```python
from build123d import *

# Parameters (mm, degrees)
SKETCH1_R           = 1.375
BOSS_EXTRUDE1_DEPTH = 1.6
CUT_EXTRUDE1_DEPTH  = 0.1
SKETCH_1_W          = 13.191380008
SKETCH_1_H          = 13.254567414
EXTRUDE_1_DEPTH     = 8
SKETCH_2_W          = 10.236154205
SKETCH_2_H          = 10.074954926
EXTRUDE_2_DEPTH     = 8


with BuildPart() as part:
    # Sketch1 → Boss-Extrude1 (new body)
    with BuildSketch(Plane.XY):
        with BuildLine():
            Line((-39.5, -28), (39.5, -28))
            ThreePointArc((39.5, -28), (41.621320344, -27.121320344), (42.5, -25))
            Line((42.5, -25), (42.5, 25))
            ThreePointArc((42.5, 25), (41.621320344, 27.121320344), (39.5, 28))
            Line((39.5, 28), (-39.5, 28))
            ThreePointArc((-39.5, 28), (-41.621320344, 27.121320344), (-42.5, 25))
            Line((-42.5, 25), (-42.5, -25))
            ThreePointArc((-42.5, -25), (-41.621320344, -27.121320344), (-39.5, -28))
        make_face()
        with Locations((-39, 24.5)):
            Circle(SKETCH1_R, mode=Mode.SUBTRACT)
        with Locations((-39, -24.5)):
            Circle(SKETCH1_R, mode=Mode.SUBTRACT)
        with Locations((19, 24.5)):
            Circle(SKETCH1_R, mode=Mode.SUBTRACT)
        with Locations((19, -24.5)):
            Circle(SKETCH1_R, mode=Mode.SUBTRACT)
    extrude(amount=BOSS_EXTRUDE1_DEPTH)

    # Sketch2 → Cut-Extrude1 (cut)
    with BuildSketch(Plane.XY.offset(1.6)):
        Polygon((-35.65, -28.636850855), (-28.15, -28.636850855), (-28.15, -23.2), (-31.573707352, -23.2), (-31.573707352, -23.3), (-28.25, -23.3), (-28.25, -28.536850855), (-35.55, -28.536850855), (-35.55, -23.3), (-32.465045999, -23.3), (-32.465045999, -23.2), (-35.65, -23.2), align=None)
        Polygon((-17.75, -17.5), (-11.015830732, -17.5), (-11.015830732, -17.6), (-17.65, -17.6), (-17.65, -33.061376344), (-3.35, -33.061376344), (-3.35, -17.6), (-9.684859924, -17.6), (-9.684859924, -17.5), (-3.25, -17.5), (-3.25, -33.161376344), (-17.75, -33.161376344), align=None)
        Polygon((0.5, -5.3), (4.5, -5.3), (4.5, -27.7), (0.5, -27.7), (0.5, -17.125), (0.6, -17.125), (0.6, -27.6), (4.4, -27.6), (4.4, -5.4), (0.6, -5.4), (0.6, -15.17398131), (0.5, -15.17398131), align=None)
        Polygon((7.5, -15.5), (9.799158316, -15.5), (9.799158316, -15.6), (7.6, -15.6), (7.6, -31.061376344), (14.4, -31.061376344), (14.4, -15.6), (12.062610562, -15.6), (12.062610562, -15.5), (14.5, -15.5), (14.5, -31.161376344), (7.5, -31.161376344), align=None)
        Polygon((-35.45, 27), (15.45, 27), (15.45, 22), (-8.906687942, 22), (-8.906687942, 22.1), (15.35, 22.1), (15.35, 26.9), (-35.35, 26.9), (-35.35, 22.1), (-11.458179647, 22.1), (-11.458179647, 22), (-35.45, 22), align=None)
        Polygon((-41.371710411, -10.514157593), (-37.371710411, -10.514157593), (-37.371710411, 0.094714316), (-37.471710411, 0.094714316), (-37.471710411, -10.414157593), (-41.271710411, -10.414157593), (-41.271710411, 10.414157593), (-37.471710411, 10.414157593), (-37.471710411, 1), (-37.371710411, 1), (-37.371710411, 10.514157593), (-41.371710411, 10.514157593), align=None)
        Polygon((23.2, -25.5), (44.7, -25.5), (44.7, -10), (23.2, -10), (23.2, -16.5), (23.3, -16.5), (23.3, -10.1), (44.6, -10.1), (44.6, -25.4), (23.3, -25.4), (23.3, -17.75), (23.2, -17.75), align=None)
        Polygon((26.8, -5.5), (54.071370237, -5.5), (54.071370237, 7.5), (26.8, 7.5), (26.8, 2.552788505), (26.9, 2.552788505), (26.9, 7.4), (53.971370237, 7.4), (53.971370237, -5.4), (26.9, -5.4), (26.9, 0.407211154), (26.8, 0.407211154), align=None)
        Polygon((26.8, 12.5), (57.71374017, 12.5), (57.71374017, 25.5), (26.8, 25.5), (26.8, 20.277341759), (26.9, 20.277341759), (26.9, 25.4), (57.61374017, 25.4), (57.61374017, 12.6), (26.9, 12.6), (26.9, 18.611308355), (26.8, 18.611308355), align=None)
    extrude(amount=-CUT_EXTRUDE1_DEPTH, mode=Mode.SUBTRACT)

    # Эскиз1 → Бобышка-Вытянуть1 (add)
    with BuildSketch(Plane.XY.offset(1.6)):
        with Locations((-13.084710258, 2.32266466)):
            Rectangle(SKETCH_1_W, SKETCH_1_H)
    extrude(amount=EXTRUDE_1_DEPTH)

    # Эскиз2 → Бобышка-Вытянуть2 (add)
    with BuildSketch(Plane.XY.offset(1.6)):
        with Locations((14.958106781, 6.145819854)):
            Rectangle(SKETCH_2_W, SKETCH_2_H)
    extrude(amount=EXTRUDE_2_DEPTH)


solid = part.part
```
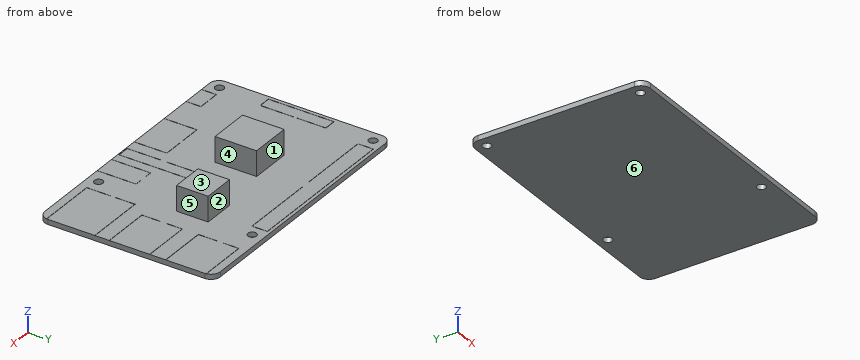
Work out the finished part from the listing and answer in its coordinate system (mm). Face numbers are marked on the shaded views. A direction names the side the tool comes from. Round coordinates to 2 decimals unless told otherwise and drop trailing zeros. Loops run counter-clockwise (first coordinate to the right, second up) from the corner with the lowest first, then second, coordinate; pieces in that order, holes last. Notation, with made-up numbers: M 64,-4.5 L 90,-4.5 A13 cw 90,6.5 Z; hole C -5,77 d7. An arc over 180 degrees is marked long. Use CSV: the item, a comma, the result in double quotes.
Q1. The mould has two halves that part along X. Classify the marked faces 4, 5 and 6: pulls with the +X half, pulls with the -X half, needs draft (parallel to the pull), parting line crosses it, or undercut.
Determined:
face 4,"undercut"
face 5,"pulls with the +X half"
face 6,"needs draft"
Q2. Section B-B, the plane y = -8.5 is taken. Determine the outline of the cut face in (x, z), then the cut area to 3 significant figures.
Determined:
outline,"M -42.5,0 L 42.5,0 L 42.5,1.6 L 4.5,1.6 L 4.5,1.5 L 4.4,1.5 L 4.4,1.6 L 0.6,1.6 L 0.6,1.5 L 0.5,1.5 L 0.5,1.6 L -37.37,1.6 L -37.37,1.5 L -37.47,1.5 L -37.47,1.6 L -41.27,1.6 L -41.27,1.5 L -41.37,1.5 L -41.37,1.6 L -42.5,1.6 Z"
area,"136 mm2"
Q3. Each of these flat-tipped pins is pushed along its axis until it touches: pin 1 (6.5 mm diameter, centred on x = 38, y = 14, fed in from +Z); pin 2 (1.5 mm diameter, centred on x = 5.5, y = -13, fed in from -Z); pin 3 (4 mm diameter, centred on x = -15, z = 7, fed in from +Y); pin 4 (2 mm diameter, centred on x = 15.5, z = 4, fed in from +Y). Where does it stop, or does it pass through?
Determined:
pin 1,"z = 1.6"
pin 2,"z = 0"
pin 3,"y = 8.95"
pin 4,"y = 11.18"
Q4. A tool of negligible diameter and unlimited length cuts with its end or side. For the marked faces 1, 2 and 3, from which of +Z, -Z, +X, -X, +Y, -Y can it reach the whole face along a straight path? Write none if from no direction.
Determined:
face 1,"+Z, -X, +Y"
face 2,"+Z, +X, -X, +Y"
face 3,"+Z, +X, -X, +Y, -Y"
Q5. Consider L1, parallel to Y at x = 19, z = 0.9 (3 decimals); L2, parallel to X at y = 6.5, z = 2.75; L3, parallel to Z at x = 29, y = 22.5. Determine where each line is inside the solid, lowest interval first.
Determined:
L1,"-28 to -25.875, -23.125 to 23.125, 25.875 to 28"
L2,"-19.68 to -6.49, 9.84 to 20.08"
L3,"0 to 1.6"
Q6. Section C-C, the plane x = -13.5 is taken. Determine the outline of the cut face in (y, z).
Determined:
outline,"M -28,0 L 28,0 L 28,1.6 L 27,1.6 L 27,1.5 L 26.9,1.5 L 26.9,1.6 L 22.1,1.6 L 22.1,1.5 L 22,1.5 L 22,1.6 L 8.95,1.6 L 8.95,9.6 L -4.3,9.6 L -4.3,1.6 L -17.5,1.6 L -17.5,1.5 L -17.6,1.5 L -17.6,1.6 L -28,1.6 Z"
Q7. Section A-A, the plane x = 19 is taken. Determine the outline of the cut face in (y, z) (3 decimals).
Determined:
outline,"M -28,0 L -25.875,0 L -25.875,1.6 L -28,1.6 Z; M -23.125,0 L 23.125,0 L 23.125,1.6 L 11.183,1.6 L 11.183,9.6 L 1.108,9.6 L 1.108,1.6 L -23.125,1.6 Z; M 25.875,0 L 28,0 L 28,1.6 L 25.875,1.6 Z"
